from build123d import *

# Parameters (mm, degrees)
F0_R     = 13.843
F1_DEPTH = 2.3622
F2_R     = 6.35


with BuildPart() as f1:
    # F0 (on Top) → F1 (new body)
    with BuildSketch(Plane.XY):
        with BuildLine():
            ThreePointArc((-18.280392, -7.3025), (-19.685, 0), (-18.280392, 7.3025))
            Line((-18.280392, 7.3025), (-34.29, 7.3025))
            Line((-34.29, 7.3025), (-34.29, -7.3025))
            Line((-34.29, -7.3025), (-18.280392, -7.3025))
        make_face()
        with BuildLine():
            ThreePointArc((18.280392, -7.3025), (19.330659, -3.718179), (19.685, 0))
            ThreePointArc((19.685, 0), (19.330659, 3.718179), (18.280392, 7.3025))
            ThreePointArc((18.280392, 7.3025), (0, 19.685), (-18.280392, 7.3025))
            ThreePointArc((-18.280392, 7.3025), (-19.685, 0), (-18.280392, -7.3025))
            ThreePointArc((-18.280392, -7.3025), (0, -19.685), (18.280392, -7.3025))
        make_face()
        Circle(F0_R, mode=Mode.SUBTRACT)
        with BuildLine():
            ThreePointArc((18.280392, 7.3025), (19.330659, 3.718179), (19.685, 0))
            ThreePointArc((19.685, 0), (19.330659, -3.718179), (18.280392, -7.3025))
            Line((18.280392, -7.3025), (76.2, -7.3025))
            Line((76.2, -7.3025), (76.2, 7.3025))
            Line((76.2, 7.3025), (18.280392, 7.3025))
        make_face()
    extrude(amount=F1_DEPTH)

    # F2
    f2_edges = [f1.edges().sort_by_distance(p)[0] for p in [
        (18.280392, -7.3025, 1.1811),
        (-18.280392, -7.3025, 1.1811),
        (-18.280392, 7.3025, 1.1811),
        (18.280392, 7.3025, 1.1811),
    ]]
    fillet(f2_edges, radius=F2_R)


solid = f1.part
Geometry check sheet. Reference: the model listing, model coordinates, mm. A direction names the side the tool comes from. Give positions to 0.01 mm unless a question says otherwise; leave off trailing zeros. Order: outer loops, then holes, each group sorted by start corner. A loop starts at its lowest first (then second) coordinate and runs counter-clockwise, first axis right, second up. Notation, with made-up numbers: (42.5, 70) - (75.5, 70) arc R19 ccw to (75.5, 103) - close; hole circle Ø5 at (16, 31). An arc over 180 degrees is marked (long way). Answer as a JSON object with one key per item and string values.
(1) Cross-section at C-C (x = 0). Record the cut outline in (y, z) (3 decimals), then the cut area to 3 significant figures.
Report:
{"outline": "(-19.685, 0) - (-13.843, 0) - (-13.843, 2.362) - (-19.685, 2.362) - close; (13.843, 0) - (19.685, 0) - (19.685, 2.362) - (13.843, 2.362) - close", "area": "27.6 mm^2"}
(2) Draft check along Y on faces 1 (the flat face through (76.2, 0, 1)), 2 (the cylindrical face through (7.4, 11.7, 1.2)), 3 (the cylindrical face through (0.281, 19.683, 1.165)), 4 (the flat face through (-28, -7.302, 1)). Enter one of: released by +Y, released by -Y, zero draft, split by the parting line, or undercut.
Report:
{"face 1": "zero draft", "face 2": "undercut", "face 3": "released by +Y", "face 4": "released by -Y"}
(3) Depth check by flat-ended pin: pin 1 Ø1 at (x, z) = (25, 0.5) entering from -Y; pin 2 Ø0.7 at (x, z) = (-28, 0.5) entering from +Y. Enter the tip coordinate at first touch or a pass-through.
Report:
{"pin 1": "y = -7.3", "pin 2": "y = 7.3"}
(4) Tool access check on faces 5 (the flat face through (-28, 7.302, 1)), 6 (the cylindrical face through (-0.281, -19.683, 1.165)), 7 (the flat face through (50, 7.302, 1)), 8 (the flat face through (20, 0, 0)), 9 (the flat face through (49, -7.302, 1)). Record the directions out of +Z, -Z, +X, -X, +Y, -Y that give a thin tool (end or side, any length) a straight path to the whole face; none if there is none.
Report:
{"face 5": "+Z, -Z, -X, +Y", "face 6": "+Z, -Z, -Y", "face 7": "+Z, -Z, +X, +Y", "face 8": "-Z, +X, -X, +Y, -Y", "face 9": "+Z, -Z, +X, -Y"}
(5) Cross-section at A-A (y = 0). Record the cut outline in (x, z).
Report:
{"outline": "(-34.29, 0) - (-13.84, 0) - (-13.84, 2.36) - (-34.29, 2.36) - close; (13.84, 0) - (76.2, 0) - (76.2, 2.36) - (13.84, 2.36) - close"}
(6) Material ranges on line 1 (X direction, y = 14, z = 1.65); line 2 (Y direction, x = -24, z = 1.5); line 3 (X direction, y = 4, z = 0.6), recorded low to high.
Report:
{"line 1": "-13.84 to 13.84", "line 2": "-7.3 to 7.3", "line 3": "-34.29 to -13.25, 13.25 to 76.2"}
(7) Cross-section at D-D (x = 69). Record the cut outline in (y, z).
Report:
{"outline": "(-7.3, 0) - (7.3, 0) - (7.3, 2.36) - (-7.3, 2.36) - close"}
